Design review of the part built by this model. Coordinates are the model's own, in mm. Face numbers are marked on the shaded views. A direction names the side the tool comes from. Coordinates: 2 decimals unless noted, no trailing zeros. Order: outer loops, then holes, each group sorted by start corner. A loop starts at its lowest first (then second) coordinate and runs counter-clockwise, first axis right, second up. Notation, with made-up numbers: (75, 81.5) -> (93, 81.5) arc R12 ccw to (93, 87.5) -> close; hole circle Ø2 at (18.5, 15.5). An arc over 180 degrees is marked (long way). Write item = value, one per line.
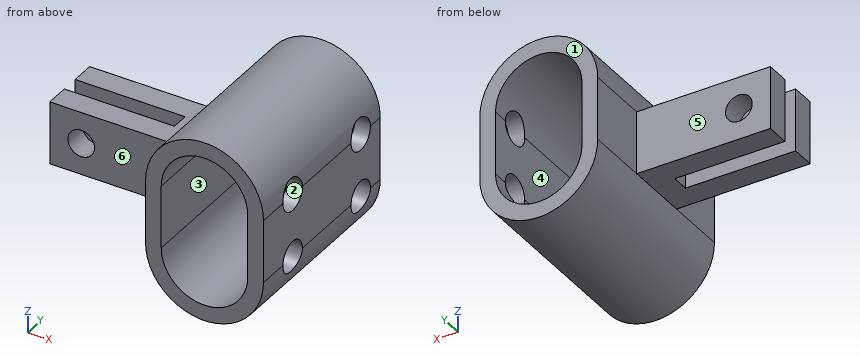
```python
from build123d import *

# Parameters (mm, degrees)
SKETCH1_W                = 6
SKETCH1_H                = 8
SKETCH1_W_2              = 8
SKETCH1_R                = 1.7
BOSS_EXTRUDE1_DEPTH      = 3
SKETCH2_W                = 8
SKETCH2_H                = 4.1
BOSS_EXTRUDE2_DEPTH      = 3
BOSS_EXTRUDE3_DEPTH      = 8
BOSS_EXTRUDE3_DEPTH_BACK = 16
SKETCH4_R                = 2
CUT_EXTRUDE1_DEPTH       = 8


with BuildPart() as part:
    # Sketch1 → Boss-Extrude1 (new body)
    with BuildSketch(Plane(origin=(0, 0, 0), x_dir=(1, 0, 0), z_dir=(0, 1, 0))):
        with Locations((7, 0)):
            Rectangle(SKETCH1_W, SKETCH1_H)
        Rectangle(SKETCH1_W_2, SKETCH1_H)
        Circle(SKETCH1_R, mode=Mode.SUBTRACT)
    extrude(amount=BOSS_EXTRUDE1_DEPTH)

    # Sketch2 → Boss-Extrude2 (add)
    with BuildSketch(Plane(origin=(10, 0, 0), x_dir=(0, 0, -1), z_dir=(1, 0, 0))):
        with Locations((0, 0.95)):
            Rectangle(SKETCH2_W, SKETCH2_H)
    extrude(amount=BOSS_EXTRUDE2_DEPTH)

    # Mirror1: part across plane


with BuildPart() as part_1:
    add(part.part)
    add(part.part.mirror(Plane(origin=(13, -1.1, 4), x_dir=(0, 0, 1), z_dir=(0, 1, 0))))

    # Sketch3 → Boss-Extrude3 (add, two sides)
    with BuildSketch(Plane(origin=(0, 3, 0), x_dir=(1, 0, 0), z_dir=(0, 1, 0))) as boss_extrude3_sk:
        with BuildLine():
            Line((28, 4), (28, -4))
            ThreePointArc((28, -4), (20.5, -11.5), (13, -4))
            Line((13, -4), (13, 4))
            ThreePointArc((13, 4), (20.5, 11.5), (28, 4))
        make_face()
        with BuildLine():
            Line((26, 4), (26, -4))
            ThreePointArc((26, -4), (20.5, -9.5), (15, -4))
            Line((15, -4), (15, 4))
            ThreePointArc((15, 4), (20.5, 9.5), (26, 4))
        make_face(mode=Mode.SUBTRACT)
    extrude(amount=BOSS_EXTRUDE3_DEPTH)
    extrude(boss_extrude3_sk.sketch, amount=-BOSS_EXTRUDE3_DEPTH_BACK)

    # Sketch4 → Cut-Extrude1 (cut)
    with BuildSketch(Plane(origin=(28, 0, 0), x_dir=(0, 0, -1), z_dir=(1, 0, 0))):
        with Locations((-4, 7)):
            Circle(SKETCH4_R)
        with Locations((4, 7)):
            Circle(SKETCH4_R)
        with Locations((4, -7)):
            Circle(SKETCH4_R)
        with Locations((-4, -7)):
            Circle(SKETCH4_R)
    extrude(amount=-CUT_EXTRUDE1_DEPTH, mode=Mode.SUBTRACT)


solid = part_1.part
```
(1) We need section A-A (x = 0). Write out the cut boundary in (y, z).
Report:
outline = (-5.2, -4) -> (-2.2, -4) -> (-2.2, -1.7) -> (-5.2, -1.7) -> close; (-5.2, 1.7) -> (-2.2, 1.7) -> (-2.2, 4) -> (-5.2, 4) -> close; (0, -4) -> (3, -4) -> (3, -1.7) -> (0, -1.7) -> close; (0, 1.7) -> (3, 1.7) -> (3, 4) -> (0, 4) -> close
(2) Insertion check: pin 1 (6.5 mm diameter, centred on y = 7, z = -0.5, fed in from -X); pin 2 (4.5 mm diameter, centred on y = -7, z = 4, fed in from -X); pin 3 (2.5 mm diameter, centred on x = 5, z = 1, fed in from +Y); pin 4 (2.5 mm diameter, centred on x = 5.5, z = 0.5, fed in from -Y). Each pin has a flat end and moves straight along its axis. Give the tip position at first contact, or say it passes through.
Report:
pin_1 = 13
pin_2 = -4
pin_3 = 3
pin_4 = -5.2
(3) The part is to be moulded in two halves that separate along Y. For the marked faces 1, 2 and 3, say which applies: released by +Y, released by -Y, zero draft, split by the parting line, or undercut.
Report:
face_1 = released by +Y
face_2 = undercut
face_3 = zero draft
(4) We need section D-D (x = 20.5). Write out the cut boundary in (y, z).
Report:
outline = (-13, -11.5) -> (11, -11.5) -> (11, -9.5) -> (-13, -9.5) -> close; (-13, 9.5) -> (11, 9.5) -> (11, 11.5) -> (-13, 11.5) -> close
(5) For L1, parallel to Y at x = 26.4, z = 4; L2, parallel to X at y = -3.2, z = 0; L3, parallel to Y at x = -3, z = 3.75, list the stretches that pass through material, from the lowest coordinate up.
Report:
L1 = -13 to -9, -5 to 5, 9 to 11
L2 = -4 to -1.7, 1.7 to 15, 26 to 28
L3 = -5.2 to -2.2, 0 to 3
(6) For the marked faces 4, 5 and 6, list the 3-axis set-ups (+Z, -Z, +X, -X, +Y, -Y) from which the entire face can be reached by the end or side of a thin tool; tool diameter is ignored.
Report:
face_4 = +Y, -Y
face_5 = +Z, -Z, -X, +Y
face_6 = +Z, -Z, -X, -Y
(7) We need section B-B (z = 0). Write out the cut boundary in (x, y).
Report:
outline = (-4, -5.2) -> (-1.7, -5.2) -> (-1.7, -2.2) -> (-4, -2.2) -> close; (-4, 0) -> (-1.7, 0) -> (-1.7, 3) -> (-4, 3) -> close; (1.7, -5.2) -> (13, -5.2) -> (13, -13) -> (15, -13) -> (15, 11) -> (13, 11) -> (13, 3) -> (1.7, 3) -> (1.7, 0) -> (10, 0) -> (10, -2.2) -> (1.7, -2.2) -> close; (26, -13) -> (28, -13) -> (28, 11) -> (26, 11) -> close
(8) We need section C-C (y = -10). Write out the cut boundary in (x, z).
Report:
outline = (13, -4) arc R7.5 ccw to (28, -4) -> (28, 4) arc R7.5 ccw to (13, 4) -> close; hole (15, -4) arc R5.5 ccw to (26, -4) -> (26, 4) arc R5.5 ccw to (15, 4) -> close
